Answer from the drawing. Dimensions are ordinates in mm from the lowest x, y and z of the part. A direction names the side the tool comes from. Round coordinates to 2 decimals unless told otherwise and drop trailing zeros. Order: outer loops, then holes, each group sorted by start corner. A loop starts at its lowest first (then second) coordinate and runs counter-clockwise, first axis right, second up. Notation, with made-up numbers: M 9.5,84 L 52.5,84 A19 cw 52.5,89 Z; hole C 20.5,39.25 d7. An arc over 180 degrees is marked long. Write item = value, one per line. Start each with the question number.
(1) A cutting plane is placed at D-D, the plane y = 24. Determine the outline of the cut face in (x, z), and give its area (3 significant figures).
(2) Each of these flat-tipped pins is pushed along its axis until it touches: pin 1 (5 mm diameter, centred on x = 10, z = 27, fed in from +Y); pin 2 (11 mm diameter, centred on x = 19.5, z = 16.5, fed in from +Y); pin 3 (5 mm diameter, centred on x = 35.5, z = 23, fed in from +Y). Where does it stop, or does it pass through?
(3) A cutting plane is placed at C-C, the plane z = 6. Determine the outline of the cut face in (x, y), and give its area (3 significant figures).
(4) A cutting plane is placed at A-A, the plane x = 16. Determine the outline of the cut face in (y, z), and give its area (3 significant figures).
(5) A cutting plane is placed at B-B, the plane y = 29. Determine the outline of the cut face in (x, z).
(6) For a pull along Z with two mould halves and no side action, classify the marked faces 3, 4, 5 and 6 as released by +Z, released by -Z, zero draft, split by the parting line, or undercut.
(7) Straight lines are drawn through the part: probe 1 along Z at (x, y) = (7.5, 22); probe 2 along X at (y, z) = (20, 2.5). For each, find the intervals that lie inside material, in ascending order. Write a range as from..to.
(8) Which of the six approach directions +Z, -Z, +X, -X, +Y, -Y give full straight-line access (tool end or side, diameter ignored) to the marked faces 1 and 2?
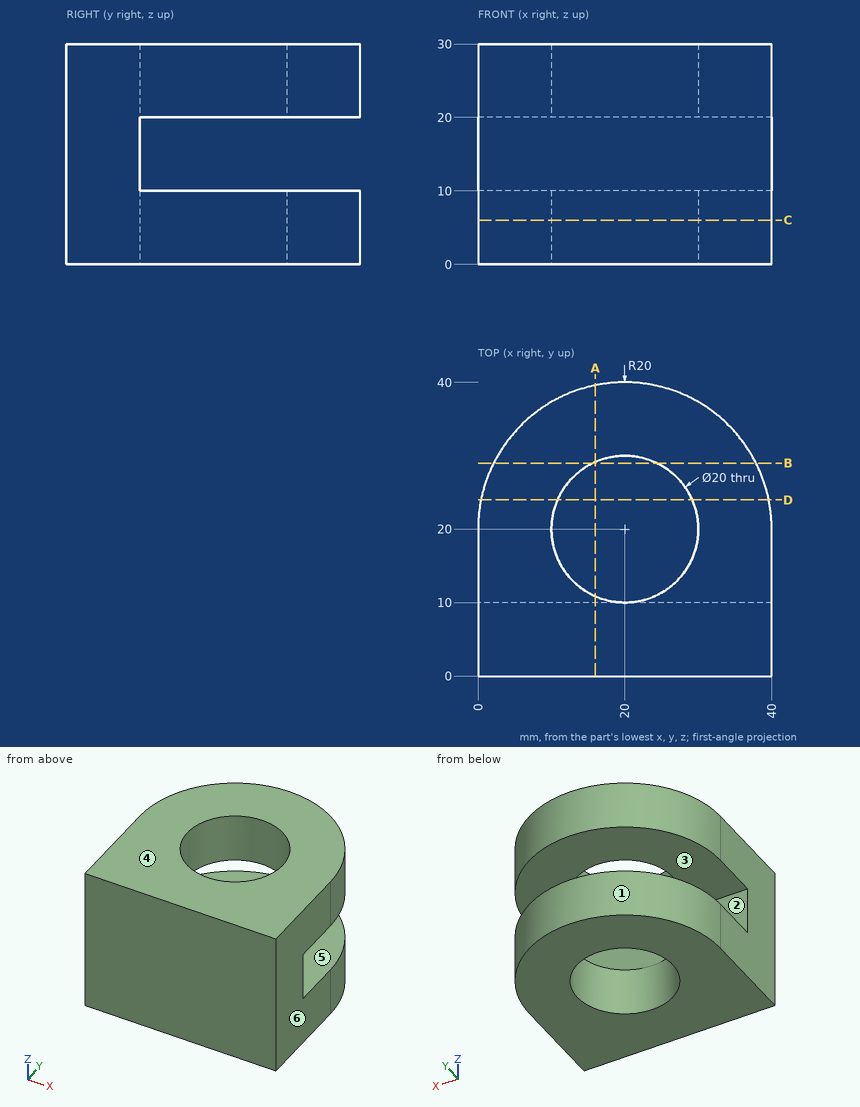
Reported:
q1.outline = M 0.4,0 L 10.83,0 L 10.83,10 L 0.4,10 Z; M 0.4,20 L 10.83,20 L 10.83,30 L 0.4,30 Z; M 29.17,0 L 39.6,0 L 39.6,10 L 29.17,10 Z; M 29.17,20 L 39.6,20 L 39.6,30 L 29.17,30 Z
q1.area = 417 mm²
q2.pin_1 = 38.54
q2.pin_2 = 40
q2.pin_3 = 35.2
q3.outline = M 0,0 L 40,0 L 40,20 A20 ccw 0,20 Z; hole C 20,20 d20
q3.area = 1,110 mm²
q4.outline = M 0,0 L 10.83,0 L 10.83,10 L 10,10 L 10,20 L 10.83,20 L 10.83,30 L 0,30 Z; M 29.17,0 L 39.6,0 L 39.6,10 L 29.17,10 Z; M 29.17,20 L 39.6,20 L 39.6,30 L 29.17,30 Z
q4.area = 525 mm²
q5.outline = M 2.14,0 L 15.64,0 L 15.64,10 L 2.14,10 Z; M 2.14,20 L 15.64,20 L 15.64,30 L 2.14,30 Z; M 24.36,0 L 37.86,0 L 37.86,10 L 24.36,10 Z; M 24.36,20 L 37.86,20 L 37.86,30 L 24.36,30 Z
q6.face_3 = undercut
q6.face_4 = released by +Z
q6.face_5 = undercut
q6.face_6 = zero draft
q7.probe_1 = 0..10, 20..30
q7.probe_2 = 0..10, 30..40
q8.face_1 = +Z, -Z, +Y
q8.face_2 = +X, -X, +Y
